Read the model definition and answer for the solid it produces. Units are mm, in the model's axes. Face numbers are marked on the shaded views. A direction names the side the tool comes from. Coordinates: 2 decimals unless noted, no trailing zeros. Order: outer loops, then holes, each group sorted by start corner. A loop starts at its lowest first (then second) coordinate and runs counter-clockwise, first axis right, second up. Notation, with made-up numbers: (68, -17) -> (78, -17) arc R37 cw to (78, 21) -> close; hole circle Ø7 at (63.25, 33.5). An arc over 180 degrees is marked (long way). Use CSV: the item, a comma, the result in double quotes.
```python
from build123d import *

# Parameters (mm, degrees)
CYLINDER009_R             = 1.9
CYLINDER009_DEPTH         = 4.5
BOX010_W                  = 45
BOX010_H                  = 10
BOX010_DEPTH              = 4.5
FILLET_R                  = 3
ARRAY002_COUNT            = 3
BOX003_W                  = 15
BOX003_H                  = 3.4
BOX003_DEPTH              = 17
ARRAY_Y_COUNT             = 2
ARRAY_Y_PITCH             = 6
CYLINDER002_R             = 2.2
CYLINDER002_DEPTH         = 6
CYLINDER001_R             = 1.9
CYLINDER001_DEPTH         = 15
FUSION001_PLACEMENT_ANGLE = 90
CYLINDER_R                = 7.5
CYLINDER_DEPTH            = 19.6
BOX002_W                  = 15
BOX002_H                  = 19.6
BOX002_DEPTH              = 12.5
CYLINDER007_R             = 15
CYLINDER007_DEPTH         = 4.5


with BuildPart() as bolt_hole002:
    # Cylinder009 → Cylinder009 (new body)
    with BuildSketch(Plane(origin=(47.6, 0, 0), x_dir=(1, 0, 0), z_dir=(0, 0, 1))):
        Circle(CYLINDER009_R)
    extrude(amount=CYLINDER009_DEPTH)


with BuildPart() as stand_stick_array:
    # Box010 → Box010 (new body)
    with BuildSketch(Plane(origin=(7.5, -5, 0), x_dir=(1, 0, 0), z_dir=(0, 0, 1))):
        with Locations((22.5, 5)):
            Rectangle(BOX010_W, BOX010_H)
    extrude(amount=BOX010_DEPTH)

    # Fillet
    fillet_edges = [stand_stick_array.edges().sort_by_distance(p)[0] for p in [
        (52.5, -5, 2.25),
        (52.5, 5, 2.25),
    ]]
    fillet(fillet_edges, radius=FILLET_R)

    # Cut006: cut bolt hole002
    add(bolt_hole002.part, mode=Mode.SUBTRACT)

    # Array002: stand stick array ×3 about axis
    array002_axis = Axis((0, 0, 0), (0, 0, 1))


with BuildPart() as stand_stick_array_1:
    add(stand_stick_array.part)
    for i in range(1, ARRAY002_COUNT):
        add(stand_stick_array.part.rotate(array002_axis, i * 360 / ARRAY002_COUNT))


with BuildPart() as side_3_extract_cube_array:
    # Box003 → Box003 (new body)
    with BuildSketch(Plane(origin=(-7.5, -7.7, 3), x_dir=(1, 0, 0), z_dir=(0, 0, 1))):
        with Locations((7.5, 1.7)):
            Rectangle(BOX003_W, BOX003_H)
    extrude(amount=BOX003_DEPTH)

    # Array Y: side 3 extract cube array ×2


with BuildPart() as side_3_extract_cube_array_1:
    add(side_3_extract_cube_array.part)
    with Locations(*[(0, i * ARRAY_Y_PITCH, 0) for i in range(1, ARRAY_Y_COUNT)]):
        add(side_3_extract_cube_array.part)


with BuildPart() as side_3_extract_cube_array_2:
    # Array placement: moved
    add(side_3_extract_cube_array_1.part.moved(Location((0, 3, 0))))


with BuildPart() as insert_hole:
    # Cylinder002 → Cylinder002 (new body)
    with BuildSketch(Plane.XY):
        Circle(CYLINDER002_R)
    extrude(amount=CYLINDER002_DEPTH)


with BuildPart() as side_3_extract_fusion:
    # Cylinder001 → Cylinder001 (new body)
    with BuildSketch(Plane.XY.offset(6)):
        Circle(CYLINDER001_R)
    extrude(amount=CYLINDER001_DEPTH)

    # Fusion001: union insert hole
    add(insert_hole.part)


with BuildPart() as side_3_extract_fusion_1:
    # Fusion001 placement: moved
    add(side_3_extract_fusion.part.moved(Location((0, 11.1, 12.5))).rotate(Axis((0, 11.1, 12.5), (1, 0, 0)), FUSION001_PLACEMENT_ANGLE))

    # Fusion002: union side 3 extract cube array
    add(side_3_extract_cube_array_2.part)


with BuildPart() as outer_cylinder:
    # Cylinder → Cylinder (new body)
    with BuildSketch(Plane(origin=(0, 11.1, 12.5), x_dir=(1, 0, 0), z_dir=(0, -1, 0))):
        Circle(CYLINDER_R)
    extrude(amount=CYLINDER_DEPTH)


with BuildPart() as side_3_cut_clone002:
    # Box002 → Box002 (new body)
    with BuildSketch(Plane(origin=(-7.5, -8.5, 0), x_dir=(1, 0, 0), z_dir=(0, 0, 1))):
        with Locations((7.5, 9.8)):
            Rectangle(BOX002_W, BOX002_H)
    extrude(amount=BOX002_DEPTH)

    # Fusion: union outer cylinder
    add(outer_cylinder.part)

    # Cut: cut side 3 extract fusion
    add(side_3_extract_fusion_1.part, mode=Mode.SUBTRACT)


with BuildPart() as side_3_cut_clone002_1:
    # Body005 placement: moved
    add(side_3_cut_clone002.part.moved(Location((0, 0, 4.5))))


with BuildPart() as stand_fusion:
    # Cylinder007 → Cylinder007 (new body)
    with BuildSketch(Plane.XY):
        Circle(CYLINDER007_R)
    extrude(amount=CYLINDER007_DEPTH)

    # Fusion007: union stand stick array, side 3 cut clone002
    add(stand_stick_array_1.part)
    add(side_3_cut_clone002_1.part)


solid = stand_fusion.part
```
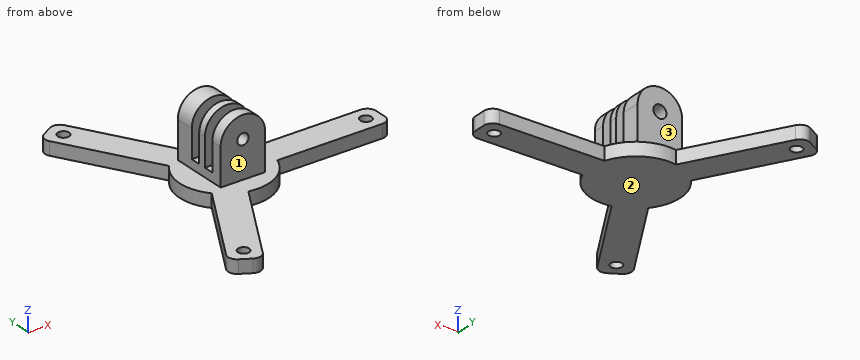
Item 1: A tool of negligible diameter and unlimited length cuts with its end or side. For the marked faces 1, 2 and 3, from which of +Z, -Z, +X, -X, +Y, -Y can it reach the whole face along a straight path? Write none if from no direction.
Return value:
face 1,"+Z, +X, -X, -Y"
face 2,"-Z, +X, -X, +Y, -Y"
face 3,"+Z, +X, -X, +Y"
Item 2: Find section C-C, the plane z = 11.5. Give the vertices of the cut face in (x, y), then the cut area to 3 significant figures.
Return value:
outline,"(-7.5, -8.5) -> (7.5, -8.5) -> (7.5, -4.7) -> (-7.5, -4.7) -> close; (-7.5, -1.3) -> (7.5, -1.3) -> (7.5, 1.3) -> (-7.5, 1.3) -> close; (-7.5, 4.7) -> (7.5, 4.7) -> (7.5, 11.1) -> (-7.5, 11.1) -> close"
area,"192 mm^2"
Item 3: Find section B-B, the plane x = 47.6. Give the vertices of the cut face in (y, z), then the cut area to 3 significant figures.
Return value:
outline,"(-5, 0) -> (-1.9, 0) -> (-1.9, 4.5) -> (-5, 4.5) -> close; (1.9, 0) -> (5, 0) -> (5, 4.5) -> (1.9, 4.5) -> close"
area,"27.9 mm^2"
Item 4: Straight lines are drawn through the part: line 1 along Y through (x, z) = (-2.5, 15.25); line 2 along Y through (x, z) = (47.6, 3.25); line 3 along Y through (x, z) = (-23.8, 1.8). For each, find the intervals that lie inside material, in ascending order.
Return value:
line 1,"y = -8.5 to -4.7, -1.3 to 1.3, 4.7 to 11.1"
line 2,"y = -5 to -1.9, 1.9 to 5"
line 3,"y = -46.76 to -43.12, -39.32 to -31.22, 31.22 to 39.32, 43.12 to 46.76"
Item 5: Find section D-D, the plane x = 0. Give the number of separate pieces and of enclosed holes in the cut face, then the cut area to 3 significant figures.
Return value:
separate pieces,"4"
enclosed holes,"0"
area,"359 mm^2"
Item 6: Each of these flat-tipped pins is pushed along its axis until it touches: P1, Ø10, axis at y = 9.5, z = 6, coming from the +X side; P2, Ø4, axis at x = 20.5, y = -3, coming from the +Z side; P3, Ø5, axis at x = 24, z = 2.5, coming from the +Y side. Where does it stop, or does it pass through?
Return value:
P1,"stops at x = 50.74"
P2,"stops at z = 4.5"
P3,"stops at y = 5"
Item 7: Find section A-A, the plane y = 0. Give the vertices of the cut face in (x, z), then the cut area to 3 significant figures.
Return value:
outline,"(-15, 0) -> (45.7, 0) -> (45.7, 4.5) -> (7.5, 4.5) -> (7.5, 17) arc R7.5 ccw to (-7.5, 17) -> (-7.5, 4.5) -> (-15, 4.5) -> close; (49.5, 0) -> (52.5, 0) -> (52.5, 4.5) -> (49.5, 4.5) -> close; hole circle Ø3.8 at (0, 17)"
area,"551 mm^2"
